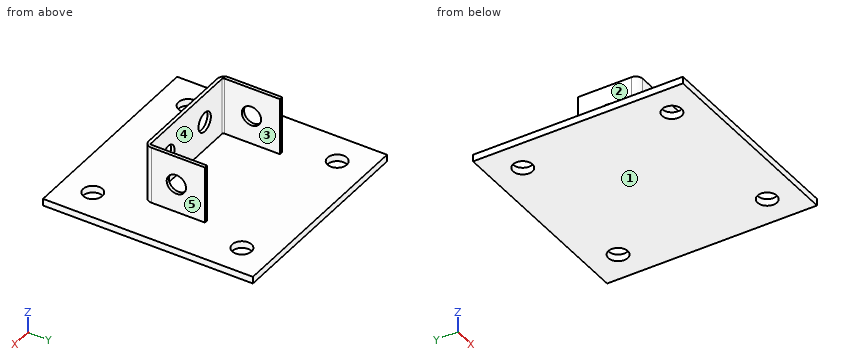
from build123d import *

# Parameters (mm, degrees)
F0_W     = 152
F0_H     = 152
F0_R     = 7
F1_DEPTH = 5
F3_DEPTH = 41.3
F4_R     = 5
F5_R     = 1
F7_D     = 14
F9_D     = 14


with BuildPart() as f1:
    # F0 (on Top) → F1 (new body)
    with BuildSketch(Plane.XY):
        Rectangle(F0_W, F0_H)
        with Locations((-54, -54)):
            Circle(F0_R, mode=Mode.SUBTRACT)
        with Locations((54, -54)):
            Circle(F0_R, mode=Mode.SUBTRACT)
        with Locations((-54, 54)):
            Circle(F0_R, mode=Mode.SUBTRACT)
        with Locations((54, 54)):
            Circle(F0_R, mode=Mode.SUBTRACT)
    extrude(amount=-F1_DEPTH)

    # F2 (on face) → F3 (join)
    with BuildSketch(Plane.XY):
        Polygon((-41.3, 20.65), (-43.8, 20.65), (-43.8, -23.15), (43.8, -23.15), (43.8, 20.65), (41.3, 20.65), (41.3, -20.65), (-41.3, -20.65), align=None)
    extrude(amount=F3_DEPTH)

    # F4
    f4_edges = [f1.edges().sort_by_distance(p)[0] for p in [
        (43.8, -23.15, 20.65),
        (-43.8, -23.15, 20.65),
    ]]
    fillet(f4_edges, radius=F4_R)

    # F5
    f5_edges = [f1.edges().sort_by_distance(p)[0] for p in [
        (41.3, -20.65, 20.65),
        (-41.3, -20.65, 20.65),
    ]]
    fillet(f5_edges, radius=F5_R)

    # F7 (through all)
    with Locations(Plane.YZ.offset(43.8)):
        with Locations((0, 20.65)):
            Hole(F7_D / 2)

    # F9 (through all)
    with Locations(Plane.XZ.offset(23.15)):
        with Locations((-20.65, 20.65), (20.65, 20.65)):
            Hole(F9_D / 2)


solid = f1.part
Input: part model. Units: mm. Frame: model coordinates. Face numbers are marked on the shaded views. A direction names the side the tool comes from. Round coordinates to 2 decimals unless told otherwise and drop trailing zeros. Order: outer loops, then holes, each group sorted by start corner. A loop starts at its lowest first (then second) coordinate and runs counter-clockwise, first axis right, second up.
1. Cut plane A-A, the plane x = 54. Output: boundary loops of the cut face in (y, z), then the cut area to 3 significant figures.
The answers:
outline: (-76, -5) - (-61, -5) - (-61, 0) - (-76, 0) - close; (-47, -5) - (47, -5) - (47, 0) - (-47, 0) - close; (61, -5) - (76, -5) - (76, 0) - (61, 0) - close
area: 620 mm2
2. Mould query, pull axis X, two halves, no side actions, for the marked faces 1, 2 and 3. Classes: released by +X, released by -X, zero draft, split by the parting line, or undercut.
The answers:
face 1: zero draft
face 2: released by -X
face 3: undercut
3. Cut plane D-D, the plane z = 20.65. Output: boundary loops of the cut face in (x, y), then the cut area to 3 significant figures.
The answers:
outline: (-43.8, -18.15) arc R5 ccw to (-38.8, -23.15) - (-27.65, -23.15) - (-27.65, -20.65) - (-40.3, -20.65) arc R1 cw to (-41.3, -19.65) - (-41.3, -7) - (-43.8, -7) - close; (-43.8, 7) - (-41.3, 7) - (-41.3, 20.65) - (-43.8, 20.65) - close; (-13.65, -23.15) - (13.65, -23.15) - (13.65, -20.65) - (-13.65, -20.65) - close; (27.65, -23.15) - (38.8, -23.15) arc R5 ccw to (43.8, -18.15) - (43.8, -7) - (41.3, -7) - (41.3, -19.65) arc R1 cw to (40.3, -20.65) - (27.65, -20.65) - close; (41.3, 7) - (43.8, 7) - (43.8, 20.65) - (41.3, 20.65) - close
area: 275 mm2
4. Cut plane C-C, the plane x = -20.65. Output: boundary loops of the cut face in (y, z).
The answers:
outline: (-76, -5) - (76, -5) - (76, 0) - (-20.65, 0) - (-20.65, 13.65) - (-23.15, 13.65) - (-23.15, 0) - (-76, 0) - close; (-23.15, 27.65) - (-20.65, 27.65) - (-20.65, 41.3) - (-23.15, 41.3) - close
5. Pin query (flat end, axial travel): P1, Ø22.5, axis at x = -20.65, z = 20.65, coming from the -Y side; P2, Ø19.5, axis at y = 9.5, z = 26.5, coming from the -X side; P3, Ø2, axis at x = -42.5, z = 10.5, coming from the +Y side. Return the tip coordinate at first contact, or that it passes through.
The answers:
P1: stops at y = -23.15
P2: stops at x = -43.8
P3: stops at y = 20.65
6. Set-up query: the marked faces 4 and 5. Return all of +Z, -Z, +X, -X, +Y, -Y with unobstructed straight access to the full face (end or side cutting, diameter ignored); none if empty.
The answers:
face 4: +Z, +Y
face 5: +Z, +X, +Y, -Y
7. Material intervals for line 1 (Y direction, x = 54, z = -3.5); line 2 (X direction, y = -7.5, z = 23); line 3 (Y direction, x = -35, z = 20), sorted ascending.
The answers:
line 1: y = -76 to -61, -47 to 47, 61 to 76
line 2: x = -43.8 to -41.3, 41.3 to 43.8
line 3: y = -23.15 to -20.65
8. Cut plane B-B, the plane y = 0. Output: boundary loops of the cut face in (x, z).
The answers:
outline: (-76, -5) - (76, -5) - (76, 0) - (43.8, 0) - (43.8, 13.65) - (41.3, 13.65) - (41.3, 0) - (-41.3, 0) - (-41.3, 13.65) - (-43.8, 13.65) - (-43.8, 0) - (-76, 0) - close; (-43.8, 27.65) - (-41.3, 27.65) - (-41.3, 41.3) - (-43.8, 41.3) - close; (41.3, 27.65) - (43.8, 27.65) - (43.8, 41.3) - (41.3, 41.3) - close
